Source: three-view drawing plus pictorial views. Frame: mm from the lowest corner of the part. A direction names the side the tool comes from. Round coordinates to 2 decimals unless told otherwise and drop trailing zeros. Order: outer loops, then holes, each group sorted by start corner. A loop starts at its lowest first (then second) coordinate and runs counter-clockwise, first axis right, second up. Notation, with made-up numbers: M 37,-37.5 L 70,-37.5 A28 cw 70,-2.5 Z; hole C -7.5,-32 d10. An arc over 180 degrees is marked long. Return JSON: item names as keys, results as strings. Group by question number.
Q1. Cut plane D-D on z = 34. Output: boundary loops of the cut face in (x, y).
Q2. Cut plane B-B on x = 44.4. Output: boundary loops of the cut face in (y, z), and give its area (3 significant figures).
Q3. Ray query, probe 1 along Y at (x, z) = (14.4, 0.5); probe 2 along X at (y, z) = (44, 17.5); probe 3 along Y at (x, z) = (87, 30). Return the intervals inside material, ascending.
Q4. Cut plane C-C on y = 15. Output: boundary loops of the cut face in (x, z).
Q5. Mould query, pull axis X, two halves, no side actions, for the marked faces 1, 2 and 3. Classes: released by +X, released by -X, zero draft, split by the parting line, or undercut.
Q6. Access query for the marked faces 4 and 5. Directions: +Z, -Z, +X, -X, +Y, -Y. A direction counts if a zero-diameter tool reaches every point of the face in a straight line with its end or side. Return the directions, or none.
Q7. Contact query for flat-ended pins moving along their axis: pin 1 (2 mm diameter, centred on x = 59.4, y = 59.98, fed in from +Z); pin 2 (19 mm diameter, centred on x = 6.5, z = 18, fed in from -Y); pin 3 (4 mm diameter, centred on x = 12.5, y = 41, fed in from +Z). Output: stop coordinate, or through.
Q8. Cut plane A-A on z = 18. Output: boundary loops of the cut face in (x, y).
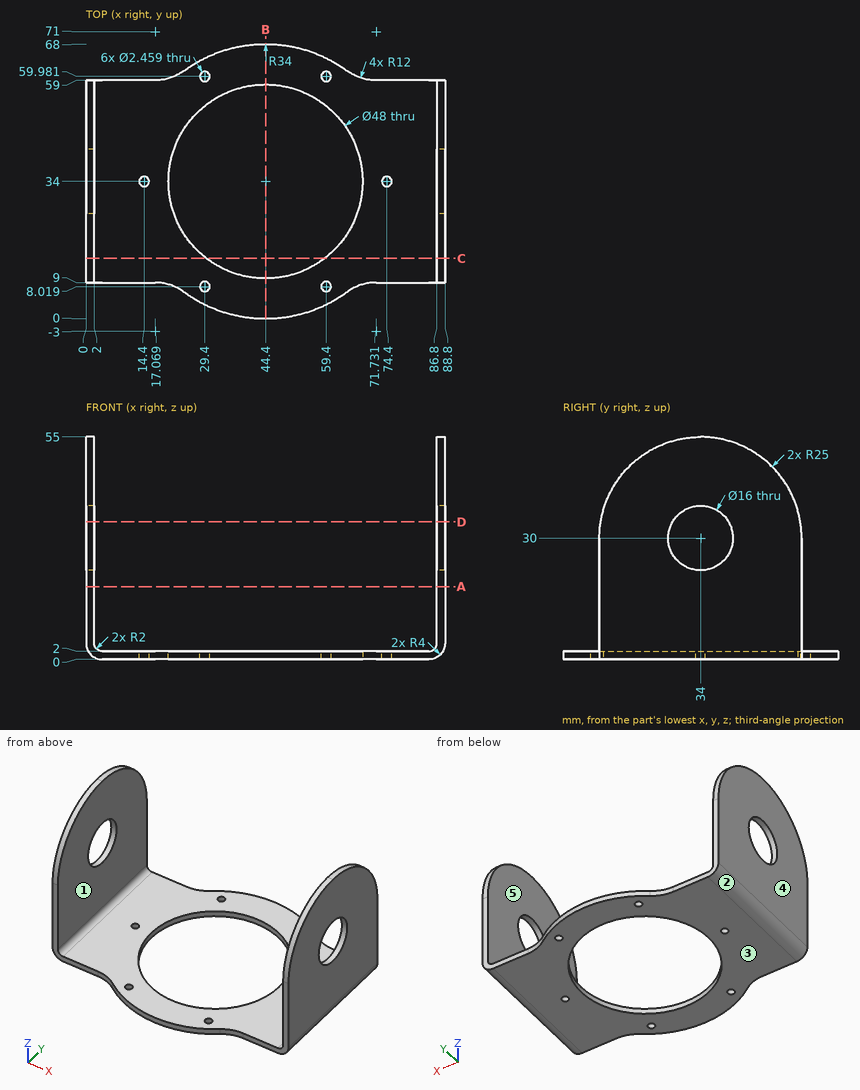
Result sheet:
{
 "1": {"outline": "M 0,9.32 L 2,9.32 L 2,27.07 L 0,27.07 Z; M 0,40.93 L 2,40.93 L 2,58.68 L 0,58.68 Z; M 86.8,9.32 L 88.8,9.32 L 88.8,27.07 L 86.8,27.07 Z; M 86.8,40.93 L 88.8,40.93 L 88.8,58.68 L 86.8,58.68 Z"},
 "2": {"outline": "M 0,0 L 10,0 L 10,2 L 0,2 Z; M 58,0 L 68,0 L 68,2 L 58,2 Z", "area": "40.0 mm²"},
 "3": {"probe 1": "y = 9 to 32.77, 35.23 to 59", "probe 2": "x = 0 to 2, 86.8 to 88.8", "probe 3": "y = 9 to 26, 42 to 59"},
 "4": {"outline": "M 0,4 A4 ccw 4,0 L 29.74,0 L 29.74,2 L 4,2 A2 cw 2,4 L 2,46.25 L 0,46.25 Z; M 59.06,0 L 84.8,0 A4 ccw 88.8,4 L 88.8,46.25 L 86.8,46.25 L 86.8,4 A2 cw 84.8,2 L 59.06,2 Z"},
 "5": {"face 1": "undercut", "face 2": "released by -X", "face 3": "zero draft"},
 "6": {"face 4": "+Z, -Z, -X, +Y, -Y", "face 5": "+Z, +Y, -Y"},
 "7": {"pin 1": "passes through", "pin 2": "stops at y = 9", "pin 3": "stops at z = 2"},
 "8": {"outline": "M 0,9 L 2,9 L 2,59 L 0,59 Z; M 86.8,9 L 88.8,9 L 88.8,59 L 86.8,59 Z"}
}
